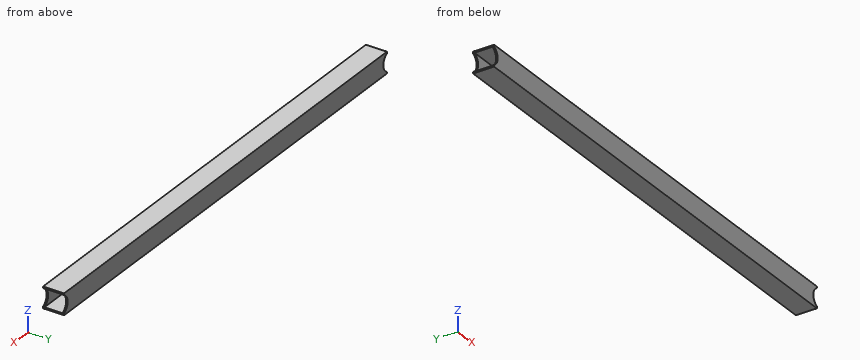
from build123d import *

# Parameters (mm, degrees)
BOSS_EXTRUDE1_DEPTH = 44.45
SKETCH3_W           = 38.1
SKETCH3_H           = 38.1
CUT_EXTRUDE1_DEPTH  = 1027.16


with BuildPart() as part:
    # Sketch2 → Boss-Extrude1 (new body)
    with BuildSketch(Plane(origin=(0, 0, 0), x_dir=(1, 0, 0), z_dir=(0, 1, 0))):
        with BuildLine():
            Line((513.08, 18.807580892), (513.08, 22.225))
            Line((513.08, 22.225), (-513.08, 22.225))
            Line((-513.08, 22.225), (-513.08, 18.807580892))
            ThreePointArc((-513.08, 18.807580892), (-504.64314077, 11.037315661), (-501.523, 0))
            ThreePointArc((-501.523, 0), (-504.64314077, -11.037315661), (-513.08, -18.807580892))
            Line((-513.08, -18.807580892), (-513.08, -22.225))
            Line((-513.08, -22.225), (513.08, -22.225))
            Line((513.08, -22.225), (513.08, -18.807580892))
            ThreePointArc((513.08, -18.807580892), (501.523, 0), (513.08, 18.807580892))
        make_face()
    extrude(amount=BOSS_EXTRUDE1_DEPTH)

    # Sketch3 → Cut-Extrude1 (cut, through all)
    with BuildSketch(Plane.ZY.offset(513.08)):
        with Locations((0, 22.225)):
            Rectangle(SKETCH3_W, SKETCH3_H)
    extrude(amount=-CUT_EXTRUDE1_DEPTH, mode=Mode.SUBTRACT)


solid = part.part
CAD build for the part. Positions are in the model's coordinates, mm. Give positions to 0.01 mm unless a question says otherwise; leave off trailing zeros. Loops run counter-clockwise (first coordinate to the right, second up) from the corner with the lowest first, then second, coordinate; pieces in that order, holes last. Notation, with made-up numbers: M 44.5,60.5 L 54.5,60.5 A20 ccw 54.5,93.5 Z; hole C -20,8.5 d2. An arc over 180 degrees is marked long. Answer in a Markdown table with one row per item. Add a question column.
Item 1: Band-saw the part on C-C on z = 12. Give the cut face in (x, y) (3 decimals), then the cut area to 3 significant figures.
Item 2: Band-saw the part on B-B on x = -249.5. Give the cut face in (y, z) (3 decimals), then the cut area to 3 significant figures.
Item 3: Drop flat-ended pins along their axis: P1, Ø12, axis at x = 338.5, z = -5.5, coming from the -Y side; P2, Ø10, axis at y = 5.5, z = -1, coming from the -X side. Give the stop position or say it passes through.
Item 4: Band-saw the part on A-A on y = 16. Give the cut face in (x, z) (3 decimals), then the cut area to 3 significant figures.
Item 5: Probe probe 1 along Y at (x, z) = (-434.5, -8) (3 decimals); probe 2 along Z at (x, y) = (-47, 26) (3 decimals); probe 3 along X at (y, z) = (42.5, -9). List the from-to ranges inside material, lowest first.
Reply:
| question | item | result |
|---|---|---|
| 1 | outline | M -505.271,0 L 505.271,0 L 505.271,3.175 L -505.271,3.175 Z; M -505.271,41.275 L 505.271,41.275 L 505.271,44.45 L -505.271,44.45 Z |
| 1 | area | 6,420 mm^2 |
| 2 | outline | M 0,-22.225 L 44.45,-22.225 L 44.45,22.225 L 0,22.225 Z; hole M 3.175,-19.05 L 41.275,-19.05 L 41.275,19.05 L 3.175,19.05 Z |
| 2 | area | 524 mm^2 |
| 3 | P1 | stops at y = 0 |
| 3 | P2 | stops at x = -502.23 |
| 4 | outline | M -513.08,-22.225 L 513.08,-22.225 L 513.08,-19.05 L -513.08,-19.05 Z; M -513.08,19.05 L 513.08,19.05 L 513.08,22.225 L -513.08,22.225 Z |
| 4 | area | 6,520 mm^2 |
| 5 | probe 1 | y = 0 to 3.175, 41.275 to 44.45 |
| 5 | probe 2 | z = -22.225 to -19.05, 19.05 to 22.225 |
| 5 | probe 3 | x = -503.54 to 503.54 |
